from build123d import *

# Parameters (mm, degrees)
BOSS_EXTRUDE4_DEPTH     = 9.525
CUT_EXTRUDE1_DEPTH      = 48.068686512
CUT_EXTRUDE1_DEPTH_BACK = 48.068686512
SKETCH6_R               = 0.635
CHAMFER2_SIZE           = 0.508
CHAMFER3_SIZE           = 0.508
SKETCH7_R               = 3.149999923
CUT_EXTRUDE2_DEPTH      = 92.200280975


with BuildPart() as part:
    # Sketch1 → Revolve1 (revolve)
    with BuildSketch(Plane.XY, mode=Mode.PRIVATE) as revolve1_sk:
        Polygon((-27.150456448, 7.9375), (-28.067, 9.525), (-28.575, 9.525), (-28.575, 4.254000001), (-38.1, 4.254000001), (-38.1, 4.000000001), (-45.1, 4.000000001), (-45.1, 1.599999975), (-35.275, 1.599999975), (-33.675000025, 0), (-28.575, 0), (0, 0), (0, 9.525), (-17.542825791, 9.525), (-18.459369343, 7.9375), (-21.634369343, 7.9375), (-22.550912895, 9.525), (-23.058912895, 9.525), (-23.975456448, 7.9375), align=None)
    revolve(revolve1_sk.sketch.rotate(Axis((-38.1, 0, 0), (1, 0, 0)), 180), axis=Axis((-38.1, 0, 0), (1, 0, 0)))

    # Sketch4 → Boss-Extrude4 (add)
    with BuildSketch(Plane.ZY.offset(28.575)):
        Polygon((0, 7.332348419), (-6.35, 3.666174209), (-6.35, -3.666174209), (0, -7.332348419), (6.35, -3.666174209), (6.35, 3.666174209), align=None)
    extrude(amount=BOSS_EXTRUDE4_DEPTH)

    # Sketch6 → Cut-Extrude1 (cut, two sides: drawn at the far end of the back side and taken through both)
    with BuildSketch(Plane.XY.offset(-CUT_EXTRUDE1_DEPTH_BACK)):
        with Locations((-25.562956448, 3.302)):
            Circle(SKETCH6_R)
        with Locations((-20.046869343, 3.302)):
            Circle(SKETCH6_R)
    extrude(amount=CUT_EXTRUDE1_DEPTH + CUT_EXTRUDE1_DEPTH_BACK, mode=Mode.SUBTRACT)

    # Chamfer2
    chamfer2_edges = [part.edges().sort_by_distance(p)[0] for p in [
        (-38.1, 0, 6.35),
        (-38.1, -5.499261314, 3.175),
        (-38.1, -5.499261314, -3.175),
        (-38.1, 0, -6.35),
        (-38.1, 5.499261314, -3.175),
        (-38.1, 5.499261314, 3.175),
    ]]
    chamfer(chamfer2_edges, length=CHAMFER2_SIZE)

    # Chamfer3
    chamfer3_edges = [part.edges().sort_by_distance(p)[0] for p in [
        (-45.1, 4.000000001, 0),
    ]]
    chamfer(chamfer3_edges, length=CHAMFER3_SIZE)

    # Mirror2: part across plane


with BuildPart() as part_1:
    add(part.part)
    add(part.part.mirror(Plane(origin=(0, 0, 0), x_dir=(0, 0, 1), z_dir=(1, 0, 0))))

    # Sketch7 → Cut-Extrude2 (cut, through all)
    with BuildSketch(Plane.ZY.offset(45.1)):
        with Locations(Location((0, 0, 0), (0, 0, 270))):
            Circle(SKETCH7_R)
    extrude(amount=-CUT_EXTRUDE2_DEPTH, mode=Mode.SUBTRACT)


solid = part_1.part
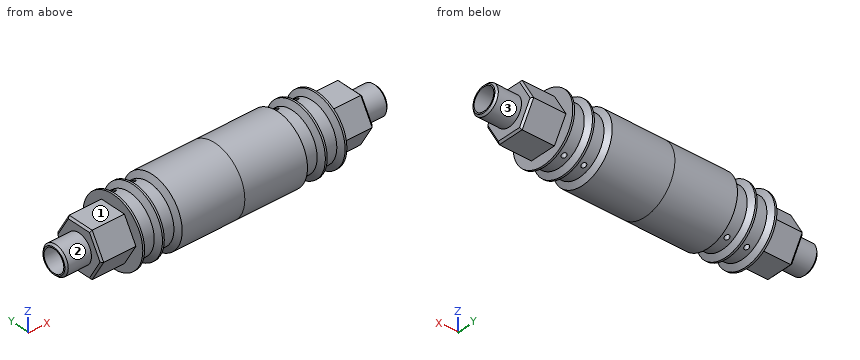
Design review of the part built by this model. Coordinates are the model's own, in mm. Face numbers are marked on the shaded views. A direction names the side the tool comes from. Round coordinates to 2 decimals unless told otherwise and drop trailing zeros. Write each loop counter-clockwise with the first axis right and the second up, starting at its lowest first coordinate (ties: lowest second). Pieces come first, ordered by that corner, then holes. Notation, with made-up numbers: M -33.5,3.5 L 22.5,3.5 A8 ccw 22.5,10.5 Z; hole C 22,79.25 d2. An arc over 180 degrees is marked long. One line per item, written item: value. Start each with the question number.
1. Take a section at B-B on z = -2. State how many separate pieces and enclosed holes the cut face has, then the cut area to 3 significant figures.
2. To check wall thickness, follow probe 1 along Z at (x, y) = (2, 0) (3 decimals); probe 2 along X at (y, z) = (4.25, 4.25); probe 3 along Y at (x, z) = (13, 1.5). State the ranges of each line that lie inside material, in increasing order. Write a range as from..to.
3. For the marked faces 1, 2 and 3, list the 3-axis set-ups (+Z, -Z, +X, -X, +Y, -Y) from which the entire face can be reached by the end or side of a thin tool; tool diameter is ignored.
4. Take a section at A-A on x = 32.5. State the section outline as (y, z) points.
5. Clearance check with flat-ended pins moving along their axes: P1, Ø4, axis at y = 5.5, z = -6.5, coming from the -X side; P2, Ø6, axis at x = 13, y = 7.5, coming from the +Z side (3 decimals); P3, Ø8, axis at x = 34.5, y = 1.5, coming from the -Z side; P4, Ø1.1, axis at x = 20.05, y = 3.3, coming from the +Z side. State where each tip first meets the part, or that it passes through.
Computed:
1. separate pieces: 2
1. enclosed holes: 4
1. area: 898 mm²
2. probe 1: z = -9.525..-3.15, 3.15..9.525
2. probe 2: x = -38.1..38.1
2. probe 3: y = -9.41..-2.77, 2.77..9.41
3. face 1: +Z, -X, +Y, -Y
3. face 2: -X
3. face 3: +X
4. outline: M -7.33,0 L -3.67,-6.35 L 3.67,-6.35 L 7.33,0 L 3.67,6.35 L -3.67,6.35 Z; hole C 0,0 d6.3
5. P1: stops at x = -37.93
5. P2: stops at z = 8.395
5. P3: stops at z = -6.35
5. P4: passes through
